from build123d import *

# Parameters (mm, degrees)
SKETCH3_W           = 40
SKETCH3_H           = 100
BOSS_EXTRUDE1_DEPTH = 20
SKETCH4_R           = 10
CUT_EXTRUDE1_DEPTH  = 104.923048454
SKETCH6_R           = 5.5
SKETCH6_R_2         = 2.1
SKETCH6_R_3         = 4.75
CUT_EXTRUDE10_DEPTH = 5
SKETCH6_2_R         = 2.1
CUT_EXTRUDE11_DEPTH = 58.445626465
FILLET1_R           = 10


with BuildPart() as part:
    # Sketch3 → Boss-Extrude1 (new body)
    with BuildSketch(Plane.XY):
        Rectangle(SKETCH3_W, SKETCH3_H)
    extrude(amount=BOSS_EXTRUDE1_DEPTH)

    # Sketch4 → Cut-Extrude1 (cut, through all)
    with BuildSketch(Plane(origin=(0, 50, 0), x_dir=(1, 0, 0), z_dir=(0, 1, 0))):
        Circle(SKETCH4_R)
    extrude(amount=-CUT_EXTRUDE1_DEPTH, mode=Mode.SUBTRACT)

    # Sketch6 → Cut-Extrude10 (cut)
    # profile 1 of 6: a face of its own
    with BuildSketch(Plane.XY.offset(20)):
        with Locations((0, 30)):
            Circle(SKETCH6_R)
        with Locations((0, 30)):
            Circle(SKETCH6_R_2, mode=Mode.SUBTRACT)
    # profile 2 of 6: a face of its own
    with BuildSketch(Plane.XY.offset(20)):
        with Locations((0, -30)):
            Circle(SKETCH6_R)
        with Locations((0, -30)):
            Circle(SKETCH6_R_2, mode=Mode.SUBTRACT)
    # profile 3 of 6: a face of its own
    with BuildSketch(Plane.XY.offset(20)):
        with Locations((-15, 30)):
            Circle(SKETCH6_R_3)
        with Locations((-15, 30)):
            Circle(SKETCH6_R_2, mode=Mode.SUBTRACT)
    # profile 4 of 6: a face of its own
    with BuildSketch(Plane.XY.offset(20)):
        with Locations((-15, -30)):
            Circle(SKETCH6_R_3)
        with Locations((-15, -30)):
            Circle(SKETCH6_R_2, mode=Mode.SUBTRACT)
    # profile 5 of 6: a face of its own
    with BuildSketch(Plane.XY.offset(20)):
        with Locations(Location((15, -30, 0), (0, 0, 180))):
            Circle(SKETCH6_R_3)
        with Locations(Location((15, -30, 0), (0, 0, 180))):
            Circle(SKETCH6_R_2, mode=Mode.SUBTRACT)
    # profile 6 of 6: a face of its own
    with BuildSketch(Plane.XY.offset(20)):
        with Locations(Location((15, 30, 0), (0, 0, 180))):
            Circle(SKETCH6_R_3)
        with Locations(Location((15, 30, 0), (0, 0, 180))):
            Circle(SKETCH6_R_2, mode=Mode.SUBTRACT)
    extrude(amount=-CUT_EXTRUDE10_DEPTH, mode=Mode.SUBTRACT)

    # Sketch6<2> → Cut-Extrude11 (cut, through all)
    with BuildSketch(Plane.XY.offset(20)):
        with Locations((0, 30)):
            Circle(SKETCH6_2_R)
        with Locations((0, -30)):
            Circle(SKETCH6_2_R)
        with Locations((-15, 30)):
            Circle(SKETCH6_2_R)
        with Locations((-15, -30)):
            Circle(SKETCH6_2_R)
        with Locations(Location((15, -30, 0), (0, 0, 180))):
            Circle(SKETCH6_2_R)
        with Locations(Location((15, 30, 0), (0, 0, 180))):
            Circle(SKETCH6_2_R)
    extrude(amount=-CUT_EXTRUDE11_DEPTH, mode=Mode.SUBTRACT)

    # Fillet1
    # the kernel refuses this fillet: 10 mm, written as the material it takes off along each edge
    with BuildSketch(Plane(origin=(-45, -50, 20), x_dir=(0, 0, -1), z_dir=(1, 0, 0))) as fillet1_piece_1:
        with BuildLine():
            CenterArc((FILLET1_R, FILLET1_R), FILLET1_R, 180, 90)
            Line((0, FILLET1_R), (0, 0))
            Line((0, 0), (FILLET1_R, 0))
        make_face()
    extrude(amount=90, mode=Mode.SUBTRACT)
    with BuildSketch(Plane(origin=(20, -75, 20), x_dir=(0, 0, -1), z_dir=(0, 1, 0))) as fillet1_piece_2:
        with BuildLine():
            CenterArc((FILLET1_R, FILLET1_R), FILLET1_R, 180, 90)
            Line((0, FILLET1_R), (0, 0))
            Line((0, 0), (FILLET1_R, 0))
        make_face()
    extrude(amount=150, mode=Mode.SUBTRACT)
    with BuildSketch(Plane(origin=(-20, 75, 20), x_dir=(1, 0, 0), z_dir=(0, -1, 0))) as fillet1_piece_3:
        with BuildLine():
            CenterArc((FILLET1_R, -FILLET1_R), FILLET1_R, 90, 90)
            Line((0, -FILLET1_R), (0, 0))
            Line((0, 0), (FILLET1_R, 0))
        make_face()
    extrude(amount=150, mode=Mode.SUBTRACT)


solid = part.part
Read the model definition and answer for the solid it produces. Units are mm, in the model's axes. A direction names the side the tool comes from. Round coordinates to 2 decimals unless told otherwise and drop trailing zeros. Order: outer loops, then holes, each group sorted by start corner. A loop starts at its lowest first (then second) coordinate and runs counter-clockwise, first axis right, second up.
1) For faces 1 (the face through (-15.46, 27.95, 7.6)), 2 (the face through (12.6, 29.9, 15)), determine the directions among +Z, -Z, +X, -X, +Y, -Y from which every point of the face is accessible in a straight line to the end or side of a thin tool.
2) The part is cut by section C-C on x = -15. Write down the section's boundary in (y, z).
3) The part is cut by section D-D on y = -42.5. Write down the section's boundary in (x, z), plus the area to 3 significant figures.
4) The mould has two halves that part along Y. Classify faces 3 (the face through (0, 6, 20)), 4 (the face through (-14.031, -31.863, 7.605)), 5 (the face through (14, -50, 5)): released by +Y, released by -Y, zero draft, split by the parting line, or undercut.
5) Flat-ended cylindrical pins translate along their axes: pin 1 (6 mm diameter, centred on y = -21, z = 14.5, fed in from -X); pin 2 (1 mm diameter, centred on x = 3.5, y = -26.5, fed in from +Z); pin 3 (6.5 mm diameter, centred on x = -16, y = 27.5, fed in from +Z); pin 4 (1 mm diameter, centred on x = -4, z = 6.5, fed in from -Y). Find the tip coordinate at first contact, or state that the pin passes through.
6) The part is cut by section B-B on z = 4.5. Write down the section's boundary in (x, y), plus the area to 3 significant figures.
7) Straight lines are drawn through the part: L1, parallel to Y at x = -15, z = 7.25; L2, parallel to Y at x = 14, z = 10.75; L3, parallel to X at y = 17, z = 8.25. For each, find the intervals that lie inside material, in ascending order.
8) The part is cut by section A-A on y = 30. Give the number of separate pieces and of enclosed holes in the cut face, plus the area to 3 significant figures.
Resolved:
1. face 1: +Z, -Z
1. face 2: +Z
2. outline: (-50, 0) - (-32.1, 0) - (-32.1, 15) - (-34.75, 15) - (-34.75, 18.66) - (-45, 18.66) arc R10 ccw to (-50, 10) - close; (-27.9, 0) - (27.9, 0) - (27.9, 15) - (25.25, 15) - (25.25, 18.66) - (-25.25, 18.66) - (-25.25, 15) - (-27.9, 15) - close; (32.1, 0) - (50, 0) - (50, 18.66) - (34.75, 18.66) - (34.75, 15) - (32.1, 15) - close
3. outline: (-20, 0) - (-10, 0) arc R10 cw to (10, 0) - (20, 0) - (20, 10) arc R10 ccw to (12.5, 19.68) - (-12.5, 19.68) arc R10 ccw to (-20, 10) - close
3. area: 593 mm2
4. face 3: zero draft
4. face 4: undercut
4. face 5: released by -Y
5. pin 1: stops at x = -19.89
5. pin 2: stops at z = 15
5. pin 3: stops at z = 19.4
5. pin 4: passes through
6. outline: (-20, -50) - (-8.93, -50) - (-8.93, 50) - (-20, 50) - close; (8.93, -50) - (20, -50) - (20, 50) - (8.93, 50) - close; hole circle Ø4.2 at (-15, -30); hole circle Ø4.2 at (-15, 30); hole circle Ø4.2 at (15, -30); hole circle Ø4.2 at (15, 30)
6. area: 2,160 mm2
7. L1: y = -50 to -32.1, -27.9 to 27.9, 32.1 to 50
7. L2: y = -49.97 to -31.85, -28.15 to 28.15, 31.85 to 50
7. L3: x = -20 to -5.65, 5.65 to 20
8. separate pieces: 4
8. enclosed holes: 0
8. area: 339 mm2
